Check sheet for the drawn part. Datum: minimum x, y, z corner. Units: mm. A direction names the side the tool comes from. Coordinates: 2 decimals unless noted, no trailing zeros. Order: outer loops, then holes, each group sorted by start corner. A loop starts at its lowest first (then second) coordinate and runs counter-clockwise, first axis right, second up. Notation, with made-up numbers: M 79.25,5 L 101.25,5 A35 ccw 101.25,42 Z; hole C 50.5,34.5 d5. An arc over 180 degrees is marked long. Use one line per item in the form item = value. Start each with the question number.
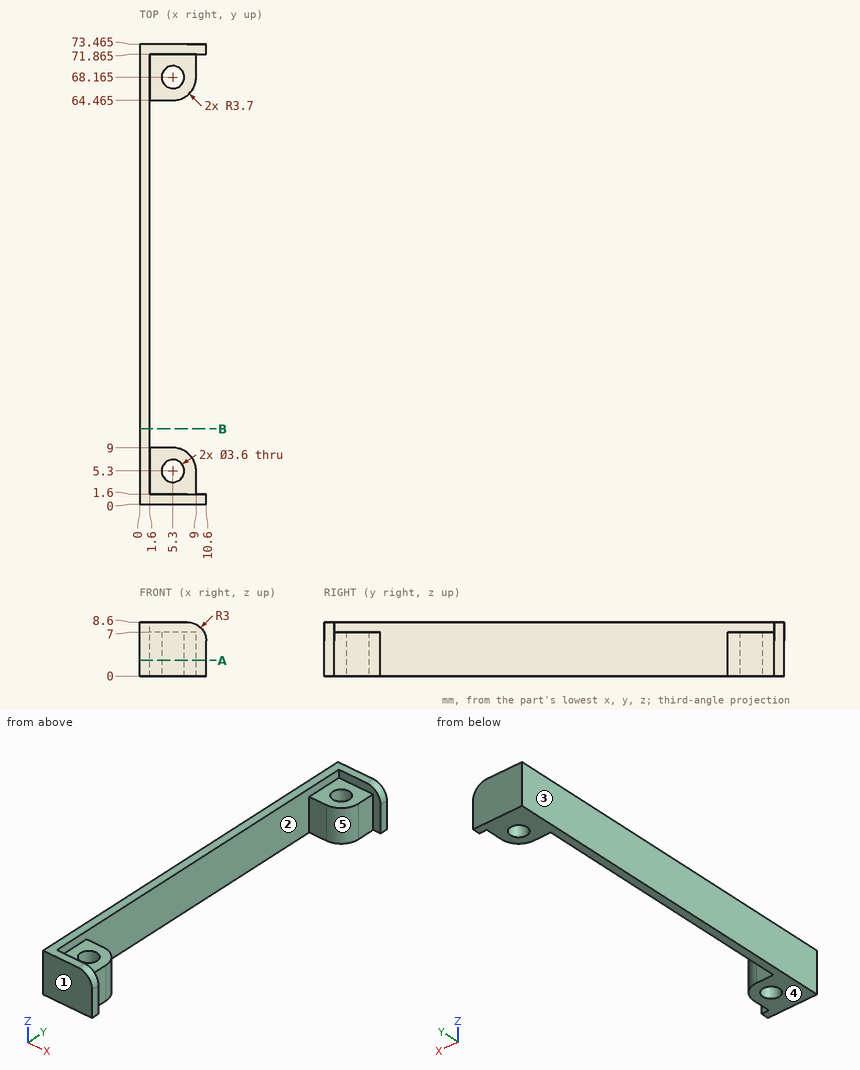
1. Release check for a two-part mould opening along Y. For the marked faces 1, 2 and 3 record: pulls with the +Y half, pulls with the -Y half, needs draft (parallel to the pull), parting line crosses it, or undercut.
2. Depth check by flat-ended pin: P1, Ø1.1, axis at y = 3, z = 5, coming from the +X side; P2, Ø2, axis at x = 3.5, y = 69.5, coming from the +Z side; P3, Ø2.5, axis at y = 36.5, z = 3.5, coming from the +X side. Enter the tip coordinate at first touch or a pass-through.
3. Cross-section at A-A on z = 2.5. Enter the section's corners in (x, y) (3 decimals), and give its area (3 significant figures).
4. Tool access check on the marked faces 4 and 5. Record the directions out of +Z, -Z, +X, -X, +Y, -Y that give a thin tool (end or side, any length) a straight path to the whole face; none if there is none.
5. Material ranges on line 1 along Y through (x, z) = (5.25, 3) (3 decimals); line 2 along Y through (x, z) = (9.5, 2) (3 decimals); line 3 along Y through (x, z) = (4, 1) (3 decimals), recorded low to high.
6. Cross-section at B-B on y = 12. Enter the section's corners in (x, z), and give its area (3 significant figures).
Final values:
q1.face_1 = pulls with the -Y half
q1.face_2 = undercut
q1.face_3 = needs draft
q2.P1 = 9
q2.P2 = 7
q2.P3 = 1.6
q3.outline = M 0,0 L 10.6,0 L 10.6,1.6 L 9,1.6 L 9,5.3 A3.7 ccw 5.3,9 L 1.6,9 L 1.6,64.465 L 5.3,64.465 A3.7 ccw 9,68.165 L 9,71.865 L 10.6,71.865 L 10.6,73.465 L 0,73.465 Z; hole C 5.3,5.3 d3.6; hole C 5.3,68.165 d3.6
q3.area = 230 mm2
q4.face_4 = -Z, +X, -X, +Y, -Y
q4.face_5 = +Z, -Z, +X
q5.line_1 = 0 to 3.501, 7.099 to 9, 64.465 to 66.366, 69.964 to 73.465
q5.line_2 = 0 to 1.6, 71.865 to 73.465
q5.line_3 = 0 to 4.055, 6.545 to 9, 64.465 to 66.92, 69.41 to 73.465
q6.outline = M 0,0 L 1.6,0 L 1.6,8.6 L 0,8.6 Z
q6.area = 13.8 mm2
